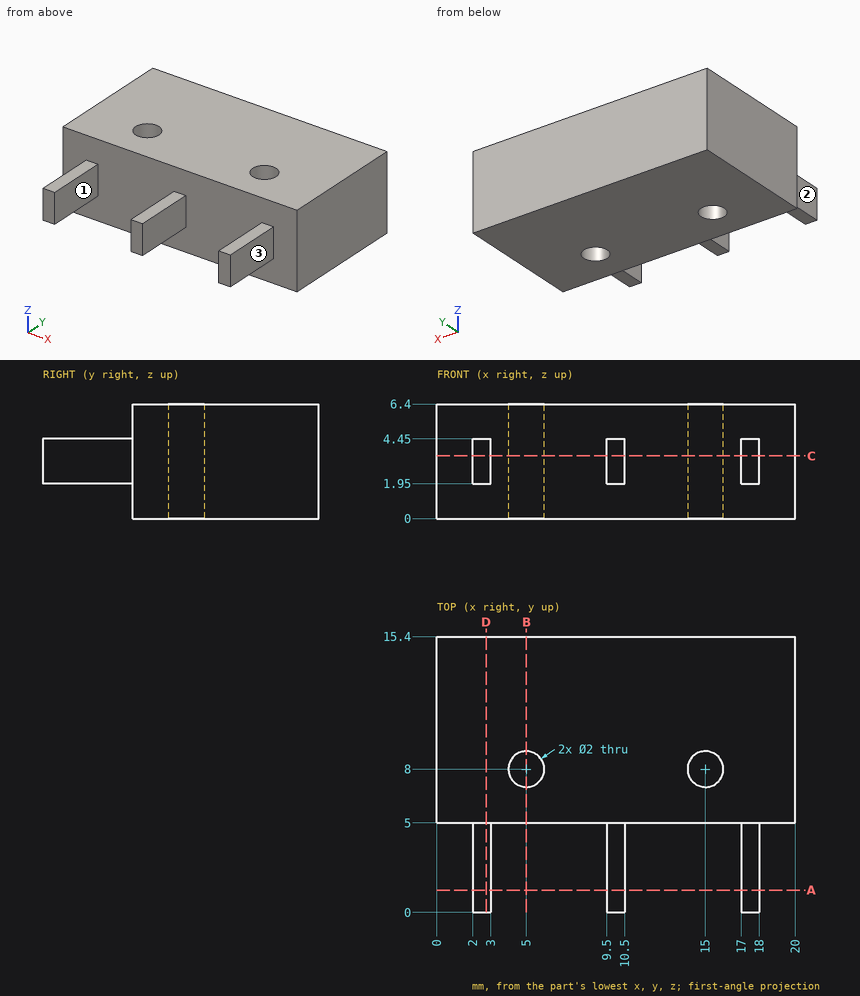
Drawing for the job (mm, zero at the part's lowest x, y, z). A direction names the side the tool comes from. Round coordinates to 2 decimals unless told otherwise and drop trailing zeros. Write each loop counter-clockwise with the first axis right and the second up, starting at its lowest first coordinate (ties: lowest second). Pieces come first, ordered by that corner, then holes. Notation, with made-up numbers: M 31.5,51 L 52.5,51 A14 cw 52.5,60 Z; hole C 4,61.25 d3. An arc over 180 degrees is marked long. Answer as a JSON object with one key per item and string values. Group by question number.
(1) Cut at D-D (x = 2.75). Give the cut face in (y, z), and give its area (3 significant figures).
(2) Cut at B-B (x = 5). Give the cut face in (y, z), and give its area (3 significant figures).
(3) Flat gauge pins, fed straight in: pin 1 (1.2 mm diameter, centred on y = 2, z = 3, fed in from +X); pin 2 (0.5 mm diameter, centred on x = 10, y = 1.5, fed in from -Z); pin 3 (0.8 mm diameter, centred on x = 17.5, y = 3.5, fed in from +Z). Where does each tip first touch, or does it go through?
(4) Which spindle directions (+Z, -Z, +X, -X, +Y, -Y) get a long thin tool onto all of the face, cutting with end or side? Do the marked faces 1, 2 and 3. Say none if no direction does.
(5) Cut at C-C (z = 3.5). Give the cut face in (x, y).
(6) Cut at A-A (y = 1.25). Give the cut face in (x, z).
(7) Drill centre lines: L1, parallel to Y at x = 15, z = 3.25; L2, parallel to Y at x = 12, z = 4.5; L3, parallel to X at y = 7.25, z = 2.5. Where is each one in solid material? Low to high.
Responses:
{
 "1": {"outline": "M 0,1.95 L 5,1.95 L 5,0 L 15.4,0 L 15.4,6.4 L 5,6.4 L 5,4.45 L 0,4.45 Z", "area": "79.1 mm2"},
 "2": {"outline": "M 5,0 L 7,0 L 7,6.4 L 5,6.4 Z; M 9,0 L 15.4,0 L 15.4,6.4 L 9,6.4 Z", "area": "53.8 mm2"},
 "3": {"pin 1": "stops at x = 18", "pin 2": "stops at z = 1.95", "pin 3": "stops at z = 4.45"},
 "4": {"face 1": "+Z, -Z, -Y", "face 2": "+Z, -Z, -X, -Y", "face 3": "+Z, -Z, +X, -Y"},
 "5": {"outline": "M 0,5 L 2,5 L 2,0 L 3,0 L 3,5 L 9.5,5 L 9.5,0 L 10.5,0 L 10.5,5 L 17,5 L 17,0 L 18,0 L 18,5 L 20,5 L 20,15.4 L 0,15.4 Z; hole C 5,8 d2; hole C 15,8 d2"},
 "6": {"outline": "M 2,1.95 L 3,1.95 L 3,4.45 L 2,4.45 Z; M 9.5,1.95 L 10.5,1.95 L 10.5,4.45 L 9.5,4.45 Z; M 17,1.95 L 18,1.95 L 18,4.45 L 17,4.45 Z"},
 "7": {"L1": "y = 5 to 7, 9 to 15.4", "L2": "y = 5 to 15.4", "L3": "x = 0 to 4.34, 5.66 to 14.34, 15.66 to 20"}
}
